Could you check a few things on this model? Use its own coordinates, in mm. A direction names the side the tool comes from. Give positions to 0.01 mm unless a question says otherwise; leave off trailing zeros. Write each loop counter-clockwise with the first axis right and the second up, starting at its lowest first coordinate (ties: lowest second). Pieces come first, ordered by that corner, then holes. Notation, with made-up numbers: (5, 53.25) - (16, 53.25) arc R17 ccw to (16, 85.25) - close; hole circle Ø10 at (42, 10.5). An arc over 180 degrees is marked (long way). Answer as CSV lines item,"result". Start each with the question number.
Q1. Imagine slicing it at D-D on y = -9. List the corners of the cut face in (x, z) for me (3 decimals), and give its area (3 significant figures).
Q2. We'd pull the mould along X, two halves only. Please class faces 6 (the face through (0, 3, -14.75)), 7 (the face through (-12.86, 8.58, 11.8)), 8 (the face through (17.286, 8.577, -0.986)), 9 (the face through (25, 8, 0)): pulls with the +X half, pulls with the -X half, needs draft (parallel to the pull), parting line crosses it, or undercut.
Q3. Imagine slicing it at B-B on y = -3. List the corners of the cut face in (x, z) for me.
Q4. If I drill on line 1 along Z through (x, y) = (16, 8.5); line 2 along Y through (x, z) = (19, -0.25); line 3 along X through (y, z) = (2, 0.5), over which ranges is the centre line in solid material (lowest first)?
Q5. Will these pins go through, and if not, where does the flat tip stop? pin 1 Ø2 at (x, y) = (-18, 9.5) entering from -Z; pin 2 Ø5 at (x, z) = (-19.5, 5.5) entering from -Y; pin 3 Ø2.5 at (x, z) = (12, 11.5) entering from +Y.
Q6. Imagine slicing it at C-C on y = 13. List the corners of the cut face in (x, z) for me, and give its area (3 significant figures).
Q7. Imagine slicing it at A-A on x = 0. List the corners of the cut face in (y, z) for me (3 decimals).
Q8. On a 3-axis mill with a long thin cutter (end or side, diameter ignored), from which of +Z, -Z, +X, -X, +Y, -Y can I reach the whole of each face in a straight line? I mean faces 1 (the face through (0.275, -6.903, -12.569)), 2 (the face through (-25, 7, 0)), 3 (the face through (0, 3, 14.75)), 4 (the face through (-11, 3, 11)), 5 (the face through (-14, -8, 0)). Say none if no direction works.
```python
from build123d import *

# Parameters (mm, degrees)
BOSS_EXTRUDE1_DEPTH = 14.75
SKETCH2_R           = 11.05
CUT_EXTRUDE1_DEPTH  = 42.744011547
SKETCH4_R           = 2.115
CUT_EXTRUDE2_DEPTH  = 12
SKETCH5_R           = 1.62
CUT_EXTRUDE3_DEPTH  = 12
CHAMFER1_SIZE       = 1
CHAMFER2_SIZE       = 0.5
CHAMFER3_SIZE       = 0.3


with BuildPart() as part:
    # Sketch1 → Boss-Extrude1 (new, symmetric)
    with BuildSketch(Plane.XY):
        Polygon((14, -15), (-14, -15), (-14, 0), (-25, 0), (-25, 15), (25, 15), (25, 0), (14, 0), align=None)
    extrude(amount=BOSS_EXTRUDE1_DEPTH, both=True)

    # Sketch2 → Cut-Extrude1 (cut, through all)
    with BuildSketch(Plane(origin=(0, 15, 0), x_dir=(1, 0, 0), z_dir=(0, 1, 0))):
        with Locations(Location((0, 0, 0), (0, 0, 180))):
            Circle(SKETCH2_R)
    extrude(amount=-CUT_EXTRUDE1_DEPTH, mode=Mode.SUBTRACT)

    # Sketch4 → Cut-Extrude2 (cut)
    with BuildSketch(Plane(origin=(0, 0, -14.75), x_dir=(-1, 0, 0), z_dir=(0, 0, -1))):
        with Locations((-17.5, 9)):
            Circle(SKETCH4_R)
        with Locations((17.5, 9)):
            Circle(SKETCH4_R)
        with Locations((0, -9)):
            Circle(SKETCH4_R)
    extrude(amount=-CUT_EXTRUDE2_DEPTH, mode=Mode.SUBTRACT)

    # Sketch5 → Cut-Extrude3 (cut)
    with BuildSketch(Plane(origin=(0, 15, 0), x_dir=(1, 0, 0), z_dir=(0, 1, 0))):
        with Locations(Location((16, 0, 0), (0, 0, 180))):
            Circle(SKETCH5_R)
        with Locations(Location((11.313708499, -11.313708499, 0), (0, 0, 180))):
            Circle(SKETCH5_R)
        with Locations(Location((-11.313708499, -11.313708499, 0), (0, 0, 180))):
            Circle(SKETCH5_R)
        with Locations(Location((-16, 0, 0), (0, 0, 180))):
            Circle(SKETCH5_R)
        with Locations(Location((-11.313708499, 11.313708499, 0), (0, 0, 180))):
            Circle(SKETCH5_R)
        with Locations(Location((11.313708499, 11.313708499, 0), (0, 0, 180))):
            Circle(SKETCH5_R)
    extrude(amount=-CUT_EXTRUDE3_DEPTH, mode=Mode.SUBTRACT)

    # Chamfer1
    chamfer1_edges = [part.edges().sort_by_distance(p)[0] for p in [
        (11.05, 15, 0),
        (17.62, 15, 0),
        (12.933708499, 15, 11.313708499),
        (-9.693708499, 15, 11.313708499),
        (-14.38, 15, 0),
        (-9.693708499, 15, -11.313708499),
        (12.933708499, 15, -11.313708499),
    ]]
    chamfer(chamfer1_edges, length=CHAMFER1_SIZE)

    # Chamfer2
    chamfer2_edges = [part.edges().sort_by_distance(p)[0] for p in [
        (19.615, 9, -14.75),
        (-15.385, 9, -14.75),
        (2.115, -9, -14.75),
    ]]
    chamfer(chamfer2_edges, length=CHAMFER2_SIZE)

    # Chamfer3
    chamfer3_edges = [part.edges().sort_by_distance(p)[0] for p in [
        (0, 15, 14.75),
        (25, 7.5, -14.75),
        (19.5, 0, -14.75),
        (-25, 7.5, 14.75),
        (14, 0, 0),
        (14, -15, 0),
        (-14, -15, 0),
        (-14, 0, 0),
        (-25, 0, 0),
        (-25, 15, 0),
        (25, 15, 0),
        (25, 0, 0),
        (-19.5, 0, 14.75),
        (-14, -7.5, 14.75),
        (0, -15, 14.75),
        (11.05, -15, 0),
        (14, -7.5, 14.75),
        (19.5, 0, 14.75),
        (25, 7.5, 14.75),
        (14, -7.5, -14.75),
        (0, -15, -14.75),
        (-14, -7.5, -14.75),
        (-19.5, 0, -14.75),
        (-25, 7.5, -14.75),
        (0, 15, -14.75),
    ]]
    chamfer(chamfer3_edges, length=CHAMFER3_SIZE)


solid = part.part
```
Conclusion:
1,outline,"(-14, -14.45) - (-13.7, -14.75) - (-2.615, -14.75) - (-2.115, -14.25) - (-2.115, -10.846) arc R11.05 cw (long way) to (2.115, -10.846) - (2.115, -14.25) - (2.615, -14.75) - (13.7, -14.75) - (14, -14.45) - (14, 14.45) - (13.7, 14.75) - (-13.7, 14.75) - (-14, 14.45) - close"
1,area,"426 mm^2"
2,face 6,"needs draft"
2,face 7,"undercut"
2,face 8,"undercut"
2,face 9,"pulls with the +X half"
3,outline,"(-14, -14.45) - (-13.7, -14.75) - (13.7, -14.75) - (14, -14.45) - (14, 14.45) - (13.7, 14.75) - (-13.7, 14.75) - (-14, 14.45) - close; hole circle Ø22.1 at (0, 0)"
4,line 1,"-2.75 to -1.62, 1.62 to 14.75"
4,line 2,"0 to 15"
4,line 3,"-25 to -11.04, 11.04 to 25"
5,pin 1,"z = -2.75"
5,pin 2,"y = 0"
5,pin 3,"y = 14.34"
6,outline,"(-25, -14.45) - (-24.7, -14.75) - (24.7, -14.75) - (25, -14.45) - (25, 14.45) - (24.7, 14.75) - (-24.7, 14.75) - (-25, 14.45) - close; hole circle Ø3.24 at (-16, 0); hole circle Ø3.24 at (-11.31, -11.31); hole circle Ø3.24 at (-11.31, 11.31); hole circle Ø22.1 at (0, 0); hole circle Ø3.24 at (11.31, -11.31); hole circle Ø3.24 at (11.31, 11.31); hole circle Ø3.24 at (16, 0)"
6,area,"1,040 mm^2"
7,outline,"(-15, -14.45) - (-14.7, -14.75) - (-11.615, -14.75) - (-11.115, -14.25) - (-11.115, -11.05) - (-14.7, -11.05) - (-15, -11.35) - close; (-15, 11.35) - (-14.7, 11.05) - (14, 11.05) - (15, 12.05) - (15, 14.45) - (14.7, 14.75) - (-14.7, 14.75) - (-15, 14.45) - close; (-6.885, -14.25) - (-6.385, -14.75) - (14.7, -14.75) - (15, -14.45) - (15, -12.05) - (14, -11.05) - (-6.885, -11.05) - close"
8,face 1,"-Z"
8,face 2,"+Z, -Z, -X, +Y, -Y"
8,face 3,"+Z, +X, -X, +Y, -Y"
8,face 4,"+Y"
8,face 5,"+Z, -Z, -X, -Y"
